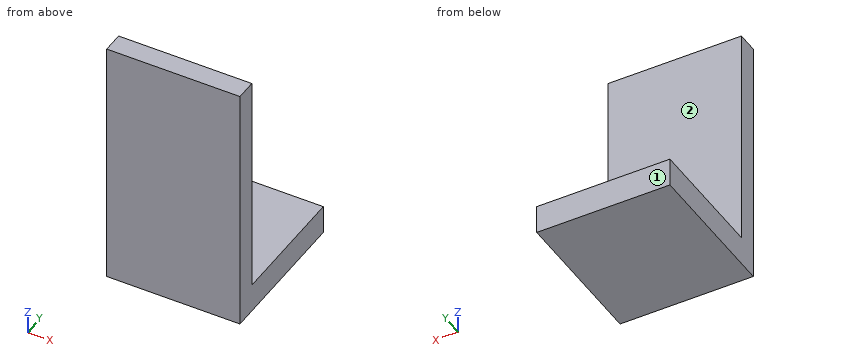
Autodesk Inventor part; units mm, degrees
ref_plane "YZ Plane" through (0, 0, 0) normal (1, 0, 0) x (0, 1, 0)
ref_plane "XZ Plane" through (0, 0, 0) normal (0, 1, 0) x (-1, 0, 0)
ref_plane "XY Plane" through (0, 0, 0) normal (0, 0, 1) x (1, 0, 0)
ref_plane "Work Plane1" through (0, 0, 0) normal (0, 0, 1) x (1, 0, 0)
sketch "Sketch1" plane through (0, 0, 0) normal (0, 0, 1) x (1, 0, 0)
  line L0 (255, -336.4839) -> (-255, -336.4839)
  line L1 (-255, -336.4839) -> (-255, 223.5161)
  line L2 (-255, 223.5161) -> (255, 223.5161)
  line L3 (255, 223.5161) -> (255, -336.4839)
  line L4 (255, -336.4839) -> (-255, 223.5161) construction
  line L5 (-255, -336.4839) -> (255, 223.5161) construction
  point P0 (0, -56.4839)
  dimension "d0" = 510
  dimension "d1" = 560
extrude "Extrusion1" add sketch "Sketch1" along normal blind 110
sketch "Sketch2" plane through (0, 0, 110) normal (0, 0, 1) x (1, 0, 0)
  line L0 (-255, -336.4839) -> (255, -336.4839)
  line L1 (255, -336.4839) -> (255, 223.5161)
  line L2 (-255, -336.4839) -> (255, -336.4839)
  line L3 (255, -336.4839) -> (255, -256.6929)
  line L4 (255, -256.6929) -> (-255, -256.6929)
  line L5 (-255, -256.6929) -> (-255, -336.4839)
  point P0 (0, 0)
extrude "Extrusion2" add sketch "Sketch2" along normal blind 860
properties part number "fotel"
Check sheet for the modelled part. Datum: model origin and axes. Units: mm. Face numbers are marked on the shaded views. A direction names the side the tool comes from. Round coordinates to 2 decimals unless told otherwise and drop trailing zeros. Write each loop counter-clockwise with the first axis right and the second up, starting at its lowest first coordinate (ties: lowest second). Pieces come first, ordered by that corner, then holes. Notation, with made-up numbers: (-15.5, 53.25) -> (19.5, 53.25) arc R6 cw to (19.5, 62.25) -> close; hole circle Ø8 at (52.5, 74). An arc over 180 degrees is marked (long way). Put each result on its own line as item: value.
(1) Sectioned sample at B-B (y = -37.5). Enter the section's corners in (x, z).
Values found:
outline: (-255, 0) -> (255, 0) -> (255, 110) -> (-255, 110) -> close
(2) Material ranges on line 1 (Z direction, x = 92, y = -133); line 2 (Y direction, x = -210, z = 738.5), recorded low to high.
Values found:
line 1: z = 0 to 110
line 2: y = -336.48 to -256.69
(3) Go/stop test with flat-tipped pins: pin 1 Ø1 at (x, z) = (81, 572.5) entering from +Y; pin 2 Ø12 at (x, y) = (-28.5, -114.5) entering from +Z. Record where each tip stops, or that it passes through.
Values found:
pin 1: stops at y = -256.69
pin 2: stops at z = 110
(4) Sectioned sample at A-A (x = 114.5). Enter the section's corners in (y, z).
Values found:
outline: (-336.48, 0) -> (223.52, 0) -> (223.52, 110) -> (-256.69, 110) -> (-256.69, 970) -> (-336.48, 970) -> close
(5) Sectioned sample at C-C (z = 718). Enter the section's corners in (x, y).
Values found:
outline: (-255, -336.48) -> (255, -336.48) -> (255, -256.69) -> (-255, -256.69) -> close
(6) Tool access check on the marked faces 1 and 2. Record the directions out of +Z, -Z, +X, -X, +Y, -Y that give a thin tool (end or side, any length) a straight path to the whole face; none if there is none.
Values found:
face 1: +Z, -Z, +X, -X, +Y
face 2: +Z, +X, -X, +Y
